Source: CAD feature listing. Evaluate the final solid. Frame: model axes, mm. A direction names the side the tool comes from. Coordinates: 2 decimals unless noted, no trailing zeros. Loops run counter-clockwise (first coordinate to the right, second up) from the corner with the lowest first, then second, coordinate; pieces in that order, holes last. Notation, with made-up numbers: M 71,85.25 L 128,85.25 A12 ccw 128,95.25 Z; hole C 69,3.5 d9. An arc over 180 degrees is marked long. One line per question, with ' | ' between items. Start each with the question number.
1. Mould query, pull axis Z, two halves, no side actions, for faces 1 (the flat face through (7, 0, 0)), 2 (the cylindrical face through (8.905, 10.042, 32.176)), 3 (the flat face through (7, 3, -24.95)), 4 (the flat face through (7, 3, 24.95)). Classes: pulls with the +Z half, pulls with the -Z half, needs draft (parallel to the pull), parting line crosses it, or undercut.
2. Section query C-C, the plane y = 3.5. Output: boundary loops of the cut face in (x, z), and give its area (4 significant figures).
3. Pin query (flat end, axial travel): P1, Ø1.5, axis at x = 3, y = 3.5, coming from the -Z side; P2, Ø3, axis at x = 11, z = 28, coming from the -Y side; P3, Ø5.5, axis at x = 8.5, y = 4, coming from the +Z side; P4, Ø2, axis at x = 7.72, z = 30.89, coming from the +Y side. Return the tip coordinate at first contact, or that it passes through.
4. Access query for faces 5 (the cylindrical face through (8.905, 10.042, -32.176)), 6 (the flat face through (8, 7, -29)), 7 (the flat face through (15, 6, 0)), 8 (the flat face through (8, 7, 29)), 9 (the flat face through (7, 12, 19.95)). Directions: +Z, -Z, +X, -X, +Y, -Y. A direction counts if a zero-diameter tool reaches every point of the face in a straight line with its end or side. Return the directions, or none.
5. Section query A-A, the plane y = 11.5. Output: boundary loops of the cut face in (x, z).
6. Ray query, probe 1 along Z at (x, y) = (8.25, 11.75); probe 2 along Y at (x, z) = (7.5, -7.5); probe 3 along Z at (x, y) = (0.5, 4). Return the intervals inside material, ascending.
7. Section query B-B, the plane x = 2.75. Output: boundary loops of the cut face in (y, z).
8. Section query D-D, the plane z = 4. Output: boundary loops of the cut face in (x, y), and give its area (4 significant figures).
```python
from build123d import *

# Parameters (mm, degrees)
SKETCH1_W           = 15
SKETCH1_H           = 49.9
BOSS_EXTRUDE1_DEPTH = 2
SKETCH2_W           = 45
SKETCH2_H           = 5
BOSS_EXTRUDE2_DEPTH = 5
SKETCH4_W           = 15
SKETCH4_H           = 49.9
BOSS_EXTRUDE3_DEPTH = 13
SKETCH5_W           = 15
SKETCH5_H           = 6
BOSS_EXTRUDE4_DEPTH = 10
SKETCH6_R           = 1.75
CUT_EXTRUDE2_DEPTH  = 48.859194519
SKETCH7_W           = 15
SKETCH7_H           = 39.9
CUT_EXTRUDE3_DEPTH  = 2.5
SKETCH8_W           = 50.368588126
SKETCH8_H           = 13
CUT_EXTRUDE4_DEPTH  = 48.859194519


with BuildPart() as part:
    # Sketch1 → Boss-Extrude1 (new body)
    with BuildSketch(Plane(origin=(0, 0, 0), x_dir=(1, 0, 0), z_dir=(0, 1, 0))):
        with Locations((7.5, 0)):
            Rectangle(SKETCH1_W, SKETCH1_H)
    extrude(amount=BOSS_EXTRUDE1_DEPTH)

    # Sketch2 → Boss-Extrude2 (add)
    with BuildSketch(Plane(origin=(0, 2, 0), x_dir=(1, 0, 0), z_dir=(0, 1, 0))):
        with Locations((-7.5, -22.45)):
            Rectangle(SKETCH2_W, SKETCH2_H)
        with Locations((-7.5, 22.45)):
            Rectangle(SKETCH2_W, SKETCH2_H)
    extrude(amount=BOSS_EXTRUDE2_DEPTH)

    # Sketch4 → Boss-Extrude3 (add)
    with BuildSketch(Plane(origin=(0, 0, 0), x_dir=(1, 0, 0), z_dir=(0, 1, 0))):
        with Locations((7.5, 0)):
            Rectangle(SKETCH4_W, SKETCH4_H)
    extrude(amount=BOSS_EXTRUDE3_DEPTH)

    # Sketch5 → Boss-Extrude4 (add)
    with BuildSketch(Plane(origin=(0, 0, -24.95), x_dir=(-1, 0, 0), z_dir=(0, 0, -1))):
        with Locations((-7.5, 10)):
            Rectangle(SKETCH5_W, SKETCH5_H)
    boss_extrude4 = extrude(amount=BOSS_EXTRUDE4_DEPTH)

    # Sketch6 → Cut-Extrude2 (cut, through all)
    with BuildSketch(Plane(origin=(0, 13, 0), x_dir=(1, 0, 0), z_dir=(0, 1, 0))):
        with Locations(Location((7.722564817, 30.885688998, 0), (0, 0, 270))):
            Circle(SKETCH6_R)
    cut_extrude2 = extrude(amount=-CUT_EXTRUDE2_DEPTH, mode=Mode.SUBTRACT)

    # Mirror1: Boss-Extrude4, Cut-Extrude2 across plane
    add(boss_extrude4.mirror(Plane.XY))
    add(cut_extrude2.mirror(Plane.XY), mode=Mode.SUBTRACT)

    # Sketch7 → Cut-Extrude3 (cut)
    with BuildSketch(Plane(origin=(0, 13, 0), x_dir=(1, 0, 0), z_dir=(0, 1, 0))):
        with Locations((7.5, 0)):
            Rectangle(SKETCH7_W, SKETCH7_H)
    extrude(amount=-CUT_EXTRUDE3_DEPTH, mode=Mode.SUBTRACT)

    # Sketch8 → Cut-Extrude4 (cut, through all)
    with BuildSketch(Plane.ZY):
        with Locations((0.234294063, 6.5)):
            Rectangle(SKETCH8_W, SKETCH8_H)
    extrude(amount=CUT_EXTRUDE4_DEPTH, mode=Mode.SUBTRACT)


solid = part.part
```
Taken from the geometry:
1) face 1: needs draft | face 2: undercut | face 3: pulls with the -Z half | face 4: pulls with the +Z half
2) outline: M 0,-24.95 L 15,-24.95 L 15,24.95 L 0,24.95 Z | area: 748.5 mm^2
3) P1: z = -24.95 | P2: y = 7 | P3: z = 24.95 | P4: through
4) face 5: +Y, -Y | face 6: -Z, +X, -X, -Y | face 7: +Z, -Z, +X, +Y, -Y | face 8: +Z, +X, -X, -Y | face 9: +X, -X, +Y
5) outline: M 0,-34.95 L 15,-34.95 L 15,-19.95 L 0,-19.95 Z; M 0,19.95 L 15,19.95 L 15,34.95 L 0,34.95 Z; hole C 7.72,-30.89 d3.5; hole C 7.72,30.89 d3.5
6) probe 1: -34.95 to -32.55, -29.22 to -19.95, 19.95 to 29.22, 32.55 to 34.95 | probe 2: 0 to 10.5 | probe 3: -24.95 to 24.95
7) outline: M 0,-24.95 L 7,-24.95 L 7,-34.95 L 13,-34.95 L 13,-19.95 L 10.5,-19.95 L 10.5,19.95 L 13,19.95 L 13,34.95 L 7,34.95 L 7,24.95 L 0,24.95 Z
8) outline: M 0,0 L 15,0 L 15,10.5 L 0,10.5 Z | area: 157.5 mm^2
